For this review, take the finished solid that the model builds, in its own axes (mm). Coordinates: 2 decimals unless noted, no trailing zeros. Order: outer loops, then holes, each group sorted by start corner. A loop starts at its lowest first (then second) coordinate and runs counter-clockwise, first axis right, second up. Notation, with made-up numbers: (-20, 1.25) -> (-3, 1.25) arc R15 cw to (-3, 22.25) -> close; hole circle Ø6 at (54.25, 72). An arc over 180 degrees is marked (long way). Answer as a JSON object with one key per item and string values. Group by question number.
1) Add section B-B, the plane x = -112. Write out the cut boundary in (y, z), then the cut area to 3 significant figures.
2) For pin 1 (7 mm diameter, centred on x = 76.67, y = -15, fed in from +Z), flat-tipped, find the tip position at first contact; note if it passes through.
3) Wall thickness on L1, parallel to X at y = -159, z = 0.1; L2, parallel to Y at x = 230, z = 0.7; L3, parallel to Y at x = -230, z = 0.8: over which ranges is each line inside the solid? List them lowest first.
4) Add section C-C, the plane x = -11.5. Write out the cut boundary in (y, z).
5) Add section A-A, the plane z = 0.55. Count the separate pieces of the cut face and the enclosed holes in it, then the cut area to 3 significant figures.
from build123d import *

# Parameters (mm, degrees)
BOSS_EXTRU_1_DEPTH      = 2
ESQUISSE3_R             = 4
ENL_V_MAT_EXTRU_1_DEPTH = 10


with BuildPart() as part:
    # Esquisse1 → Boss.-Extru.1 (new body)
    with BuildSketch(Plane.XY):
        Polygon((-250, 0), (250, 0), (250, -563), (-250, -460), align=None)
    extrude(amount=BOSS_EXTRU_1_DEPTH)

    # Esquisse3 → Enlèv. mat.-Extru.1 (cut)
    with BuildSketch(Plane(origin=(0, 0, 0), x_dir=(-1, 0, 0), z_dir=(0, 0, -1))):
        with Locations((-230, -15)):
            Circle(ESQUISSE3_R)
        with Locations((-76.666666667, -15)):
            Circle(ESQUISSE3_R)
        with Locations((76.666666667, -15)):
            Circle(ESQUISSE3_R)
        with Locations((230, -15)):
            Circle(ESQUISSE3_R)
        with Locations((230, -159.60167891)):
            Circle(ESQUISSE3_R)
        with Locations((230, -304.203357819)):
            Circle(ESQUISSE3_R)
        with Locations((76.666666667, -480.391703395)):
            Circle(ESQUISSE3_R)
        with Locations((-76.666666667, -511.978370062)):
            Circle(ESQUISSE3_R)
        with Locations((-230, -543.565036729)):
            Circle(ESQUISSE3_R)
        with Locations((-230, -367.376691152)):
            Circle(ESQUISSE3_R)
        with Locations((-230, -191.188345576)):
            Circle(ESQUISSE3_R)
        with Locations((230, -448.805036729)):
            Circle(ESQUISSE3_R)
    extrude(amount=-ENL_V_MAT_EXTRU_1_DEPTH, mode=Mode.SUBTRACT)


solid = part.part
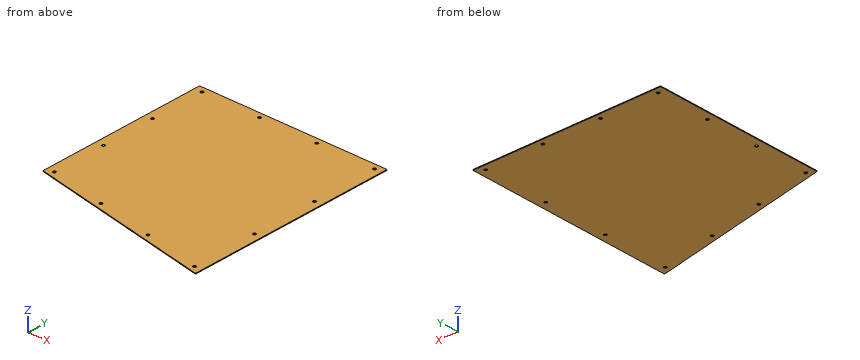
Output values:
{
 "1": {"outline": "(-488.43, 0) -> (0, 0) -> (0, 2) -> (-488.43, 2) -> close", "area": "977 mm²"},
 "2": {"pin 1": "passes through"},
 "3": {"L1": "x = -250 to -233.95, -226.05 to 250", "L2": "y = -558.88 to -547.57, -539.57 to -371.38, -363.38 to -195.19, -187.19 to -19, -11 to 0", "L3": "y = -464.12 to -452.81, -444.81 to -308.2, -300.2 to -163.6, -155.6 to -19, -11 to 0"},
 "4": {"outline": "(-509.13, 0) -> (0, 0) -> (0, 2) -> (-509.13, 2) -> close"},
 "5": {"separate pieces": "1", "enclosed holes": "12", "area": "255,000 mm²"}
}
